Part model, mm, in its own coordinate system. Face numbers are marked on the shaded views. Round coordinates to 2 decimals unless told otherwise and drop trailing zeros. Write each loop counter-clockwise with the first axis right and the second up, starting at its lowest first coordinate (ties: lowest second). Pieces come first, ordered by that corner, then holes. Notation, with made-up numbers: (59, 31.5) -> (96, 31.5) arc R33 ccw to (96, 63.5) -> close; hole circle Ø6 at (19, 58). An arc over 180 degrees is marked (long way). Return JSON: item names as keys, results as strings. Group by question number.
(1) Drop flat-ended pins along their axis: pin 1 Ø2 at (x, z) = (64, -56.5) entering from -Y; pin 2 Ø1.5 at (x, y) = (21.5, -41) entering from +Z; pin 3 Ø1.5 at (x, z) = (98, -13.5) entering from +Y. Give the stop position or say it passes through.
(2) Saw through at D-D (x = 16.5). List the corners of the cut face in (y, z).
(3) Saw through at B-B (x = 55.5). List the corners of the cut face in (y, z), plus the area to 3 significant figures.
(4) Mould opens along Z. For the marked faces 1 and 2 say: +Z half, -Z half, draft (parallel to the pull), parting line (faces both ways), or undercut.
(5) Saw through at A-A (y = -20). List the corners of the cut face in (x, z).
(6) Drill centre lines: L1, parallel to Z at x = 67, y = -31; L2, parallel to Y at x = 66.5, z = 385; L3, parallel to Z at x = 92, y = -118. Where is each one in solid material? Low to high. Write a range as from..to.
(7) Saw through at C-C (z = -82.5). List the corners of the cut face in (x, y), plus the area to 3 significant figures.
from build123d import *

# Parameters (mm, degrees)
FILLET1_R = 31.75


with BuildPart() as part:
    # Sweep2: sweep along a path in Sketch1
    with BuildLine(Plane(origin=(0, 0, 0), x_dir=(0, 0, -1), z_dir=(1, 0, 0))) as sweep2_path:
        Line((-430.75225, -177.8635), (-430.75225, 0))
        Line((-430.75225, 0), (430.75225, 0))
        Line((430.75225, 0), (430.75225, -177.8635))
    # Sketch2 → Sweep2 (sweep)
    with BuildSketch(Plane(origin=(0, 0, 0), x_dir=(1, 0, 0), z_dir=(0, 1, 0))):
        with BuildLine():
            Line((0, -430.75225), (114.3, -430.75225))
            Line((114.3, -430.75225), (114.3, -462.50225))
            ThreePointArc((114.3, -462.50225), (105.000640303, -484.952890303), (82.55, -494.25225))
            Line((82.55, -494.25225), (31.75, -494.25225))
            ThreePointArc((31.75, -494.25225), (9.299359697, -484.952890303), (0, -462.50225))
            Line((0, -462.50225), (0, -430.75225))
        make_face()
    sweep(path=sweep2_path.line, transition=Transition.RIGHT)

    # Fillet1
    # the kernel refuses this fillet: 31.75 mm, written as the material it takes off along each edge
    with BuildSketch(Plane(origin=(82.55, 31.75, -462.50225), x_dir=(0, 0, -1), z_dir=(0, 1, 0))) as fillet1_piece_1_section:
        Polygon((0, 0), (FILLET1_R * 1.02, 0), (FILLET1_R * 1.02, -FILLET1_R * 1.02), (0, -FILLET1_R * 1.02), align=None)
    fillet1_piece_1 = extrude(amount=FILLET1_R * 1.02, mode=Mode.PRIVATE)
    fillet1_piece_1 = fillet1_piece_1 - Plane(origin=(82.55, 31.75, -462.50225), x_dir=(-0.7071067811865477, 0, 0.7071067811865474), z_dir=(0, 1, 0)) * Sphere(FILLET1_R, mode=Mode.PRIVATE)
    add(fillet1_piece_1, mode=Mode.SUBTRACT)
    with BuildSketch(Plane(origin=(31.75, 31.75, -462.50225), x_dir=(0, 0, -1), z_dir=(0, 1, 0))) as fillet1_piece_2_section:
        Polygon((0, 0), (FILLET1_R * 1.02, 0), (FILLET1_R * 1.02, FILLET1_R * 1.02), (0, FILLET1_R * 1.02), align=None)
    fillet1_piece_2 = extrude(amount=FILLET1_R * 1.02, mode=Mode.PRIVATE)
    fillet1_piece_2 = fillet1_piece_2 - Plane(origin=(31.75, 31.75, -462.50225), x_dir=(0.7071067811865475, 0, 0.7071067811865475), z_dir=(0, 1, 0)) * Sphere(FILLET1_R, mode=Mode.PRIVATE)
    add(fillet1_piece_2, mode=Mode.SUBTRACT)
    with BuildSketch(Plane(origin=(31.75, 31.75, 462.50225), x_dir=(0, 1, 0), z_dir=(0, 0, 1))) as fillet1_piece_3_section:
        Polygon((0, 0), (FILLET1_R * 1.02, 0), (FILLET1_R * 1.02, FILLET1_R * 1.02), (0, FILLET1_R * 1.02), align=None)
    fillet1_piece_3 = extrude(amount=FILLET1_R * 1.02, mode=Mode.PRIVATE)
    fillet1_piece_3 = fillet1_piece_3 - Plane(origin=(31.75, 31.75, 462.50225), x_dir=(0.7071067811865477, -0.7071067811865475, 0), z_dir=(0, 0, 1)) * Sphere(FILLET1_R, mode=Mode.PRIVATE)
    add(fillet1_piece_3, mode=Mode.SUBTRACT)
    with BuildSketch(Plane(origin=(82.55, 31.75, 462.50225), x_dir=(0, 1, 0), z_dir=(0, 0, 1))) as fillet1_piece_4_section:
        Polygon((0, 0), (FILLET1_R * 1.02, 0), (FILLET1_R * 1.02, -FILLET1_R * 1.02), (0, -FILLET1_R * 1.02), align=None)
    fillet1_piece_4 = extrude(amount=FILLET1_R * 1.02, mode=Mode.PRIVATE)
    fillet1_piece_4 = fillet1_piece_4 - Plane(origin=(82.55, 31.75, 462.50225), x_dir=(-0.7071067811865475, -0.7071067811865476, 0), z_dir=(0, 0, 1)) * Sphere(FILLET1_R, mode=Mode.PRIVATE)
    add(fillet1_piece_4, mode=Mode.SUBTRACT)
    with BuildSketch(Plane(origin=(82.55, 63.5, -494.25225), x_dir=(0, 0, 1), z_dir=(-1, 0, 0)), Plane(origin=(82.55, 63.5, 494.25225), x_dir=(0, -1, 0), z_dir=(-1, 0, 0))) as fillet1_piece_5:
        with BuildLine():
            CenterArc((FILLET1_R, -FILLET1_R), FILLET1_R, 90, 90)
            Line((0, -FILLET1_R), (0, 0))
            Line((0, 0), (FILLET1_R, 0))
        make_face()
    extrude(amount=50.8, mode=Mode.SUBTRACT)


solid = part.part
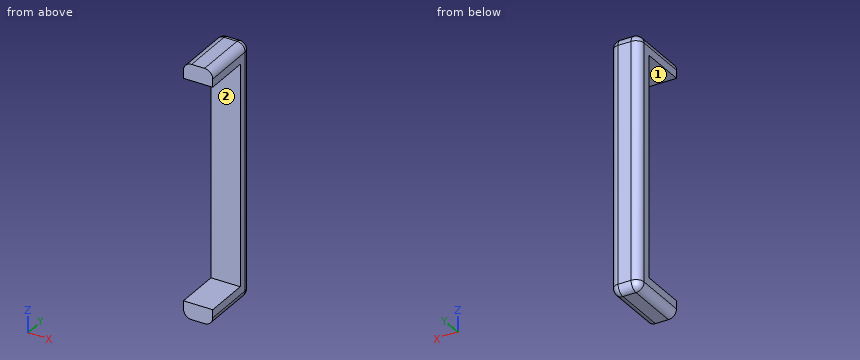
Computed values:
{
 "1": {"pin 1": "y = 0", "pin 2": "z = 492.8", "pin 3": "y = 59.89"},
 "2": {"outline": "(-177.86, -490.35) -> (31.75, -490.35) arc R27.85 ccw to (59.6, -462.5) -> (59.6, 462.5) arc R27.85 ccw to (31.75, 490.35) -> (-177.86, 490.35) -> (-177.86, 430.75) -> (0, 430.75) -> (0, -430.75) -> (-177.86, -430.75) -> close"},
 "3": {"outline": "(-177.86, -494.25) -> (31.75, -494.25) arc R31.75 ccw to (63.5, -462.5) -> (63.5, 462.5) arc R31.75 ccw to (31.75, 494.25) -> (-177.86, 494.25) -> (-177.86, 430.75) -> (0, 430.75) -> (0, -430.75) -> (-177.86, -430.75) -> close", "area": "84,900 mm2"},
 "4": {"face 1": "undercut", "face 2": "undercut"},
 "5": {"outline": "(0, -462.5) arc R31.75 ccw to (31.75, -494.25) -> (82.55, -494.25) arc R31.75 ccw to (114.3, -462.5) -> (114.3, -430.75) -> (0, -430.75) -> close; (0, 430.75) -> (114.3, 430.75) -> (114.3, 462.5) arc R31.75 ccw to (82.55, 494.25) -> (31.75, 494.25) arc R31.75 ccw to (0, 462.5) -> close"},
 "6": {"L1": "-494.25..-430.75, 430.75..494.25", "L2": "0..63.5", "L3": "-492.81..-430.75, 430.75..492.81"},
 "7": {"outline": "(0, 0) -> (114.3, 0) -> (114.3, 31.75) arc R31.75 ccw to (82.55, 63.5) -> (31.75, 63.5) arc R31.75 ccw to (0, 31.75) -> close", "area": "6,830 mm2"}
}
